Geometry: final body of the model. Coordinates: model frame, mm. Face numbers are marked on the shaded views. Give positions to 0.01 mm unless a question says otherwise; leave off trailing zeros. Write each loop counter-clockwise with the first axis right and the second up, starting at its lowest first coordinate (ties: lowest second). Pieces come first, ordered by that corner, then holes.
```python
from build123d import *

# Parameters (mm, degrees)
SKETCH_1_R               = 10
EXTRUDE_1_DEPTH          = 10
EXTRUDE_2_DEPTH          = 10
CUT_EXTRUDE_2_DEPTH      = 81.925892025
CUT_EXTRUDE_2_DEPTH_BACK = 81.925892025
SKETCH_3_R               = 3
CUT_EXTRUDE_3_DEPTH      = 82.240384046
CUT_EXTRUDE_3_DEPTH_BACK = 82.240384046
SKETCH_7_W               = 6
SKETCH_7_H               = 16
CUT_EXTRUDE_4_DEPTH      = 82.240384046
CUT_EXTRUDE_4_DEPTH_BACK = 82.240384046
SKETCH_8_R               = 2
CHAMFER_1_SIZE           = 1
CHAMFER_2_SIZE           = 0.5


with BuildPart() as part:
    # 草图1 → 凸台-拉伸1 (new body)
    with BuildSketch(Plane.XY):
        Circle(SKETCH_1_R)
    extrude(amount=EXTRUDE_1_DEPTH)

    # 草图2 → 凸台-拉伸2 (add)
    with BuildSketch(Plane.XY):
        with BuildLine():
            Line((-9.980372744, -0.626226703), (-5, -80))
            Line((-5, -80), (5, -80))
            Line((5, -80), (9.980372744, -0.626226703))
            ThreePointArc((9.980372744, -0.626226703), (0, -10), (-9.980372744, -0.626226703))
        make_face()
    extrude(amount=EXTRUDE_2_DEPTH)

    # 草图3 → 切除-拉伸2 (cut, two sides: drawn at the far end of the back side and taken through both)
    with BuildSketch(Plane(origin=(0, 0, 3), x_dir=(-1, 0, 0), z_dir=(0, 0, -1)).offset(-CUT_EXTRUDE_2_DEPTH_BACK)):
        Circle(SKETCH_3_R)
    extrude(amount=CUT_EXTRUDE_2_DEPTH + CUT_EXTRUDE_2_DEPTH_BACK, mode=Mode.SUBTRACT)

    # 草图7 → 切除-拉伸3 (cut, two sides: drawn at the far end of the back side and taken through both)
    with BuildSketch(Plane(origin=(0, 0, 0), x_dir=(0, 0, -1), z_dir=(1, 0, 0)).offset(-CUT_EXTRUDE_3_DEPTH_BACK)):
        with Locations((-5, -76)):
            Rectangle(SKETCH_7_W, SKETCH_7_H)
    extrude(amount=CUT_EXTRUDE_3_DEPTH + CUT_EXTRUDE_3_DEPTH_BACK, mode=Mode.SUBTRACT)

    # 草图8 → 切除-拉伸4 (cut, two sides: drawn at the far end of the back side and taken through both)
    with BuildSketch(Plane.XY.offset(10).offset(-CUT_EXTRUDE_4_DEPTH_BACK)):
        with Locations((0, -74)):
            Circle(SKETCH_8_R)
    extrude(amount=CUT_EXTRUDE_4_DEPTH + CUT_EXTRUDE_4_DEPTH_BACK, mode=Mode.SUBTRACT)

    # 倒角1
    chamfer_1_edges = [part.edges().sort_by_distance(p)[0] for p in [
        (3, 0, 10),
    ]]
    chamfer(chamfer_1_edges, length=CHAMFER_1_SIZE)

    # 倒角2
    chamfer_2_edges = [part.edges().sort_by_distance(p)[0] for p in [
        (-2, -74, 10),
        (-2, -74, 8),
        (-2, -74, 0),
        (-2, -74, 2),
    ]]
    chamfer(chamfer_2_edges, length=CHAMFER_2_SIZE)


solid = part.part
```
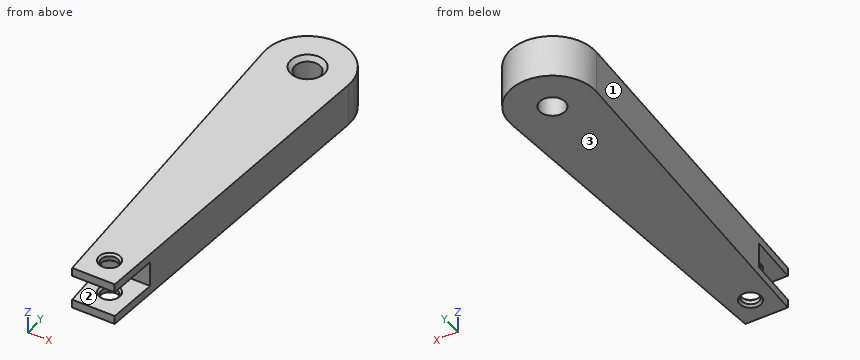
Item 1: Line query: L1, parallel to Y at x = 0, z = 0.9; L2, parallel to Z at x = 4.75, y = -75.5; L3, parallel to Y at x = 0, z = 6.75. Output: solid intervals per line, ascending.
Found:
L1: y = -80 to -76, -72 to -3, 3 to 10
L2: z = 0 to 2, 8 to 10
L3: y = -68 to -3, 3 to 10
Item 2: Section A-A, the plane x = 0. State how many separate pieces and enclosed holes the cut face has, plus the area to 3 significant figures.
Found:
separate pieces: 4
enclosed holes: 0
area: 750 mm2
Item 3: Section B-B, the plane z = 6.25. Return the cut outline in (x, y).
Found:
outline: (-9.98, -0.63) - (-5.75, -68) - (5.75, -68) - (9.98, -0.63) arc R10 ccw (long way) to start; hole circle Ø6 at (0, 0)
Item 4: Pin query (flat end, axial travel): pin 1 Ø4.5 at (x, y) = (0, -74) entering from -Z; pin 2 Ø5 at (y, z) = (-49.5, 8) entering from +X; pin 3 Ø3 at (x, z) = (-7, 5.5) entering from -Y. Return the tip coordinate at first contact, or that it passes through.
Found:
pin 1: stops at z = 0.25
pin 2: stops at x = 7.07
pin 3: stops at y = -68
Item 5: Pull-direction query (Z, two-part tool) for the marked faces 1, 2 and 3; classes: +Z half, -Z half, draft (parallel to the pull), parting line (faces both ways), or undercut.
Found:
face 1: draft
face 2: undercut
face 3: -Z half
Item 6: Section D-D, the plane x = 8.25. Return the cut outline in (y, z), plus the area to 3 significant figures.
Found:
outline: (-28.2, 0) - (5.65, 0) - (5.65, 10) - (-28.2, 10) - close
area: 339 mm2
Item 7: Section C-C, the plane y = -74. Return the cut outline in (x, z).
Found:
outline: (-5.38, 0) - (-2.5, 0) - (-2, 0.5) - (-2, 1.5) - (-2.5, 2) - (-5.38, 2) - close; (-5.38, 8) - (-2.5, 8) - (-2, 8.5) - (-2, 9.5) - (-2.5, 10) - (-5.38, 10) - close; (2, 0.5) - (2.5, 0) - (5.38, 0) - (5.38, 2) - (2.5, 2) - (2, 1.5) - close; (2, 8.5) - (2.5, 8) - (5.38, 8) - (5.38, 10) - (2.5, 10) - (2, 9.5) - close
